Read the model definition and answer for the solid it produces. Units are mm, in the model's axes. Coordinates: 2 decimals unless noted, no trailing zeros. Write each loop counter-clockwise with the first axis right and the second up, starting at its lowest first coordinate (ties: lowest second). Pieces come first, ordered by that corner, then holes.
(1) Straight lines are drawn through the part: line 1 along X through (y, z) = (-19, 14.25); line 2 along Y through (x, z) = (100.5, 24.25). For each, find the intervals that lie inside material, in ascending order.
(2) The part is cut by section B-B, the plane x = 265. Determine the outline of the cut face in (y, z), and give its area (3 significant figures).
(3) The part is cut by section A-A, the plane y = 456.5. Determine the outline of the cut face in (x, z).
(4) The part is cut by section C-C, the plane z = 4.75. Determine the outline of the cut face in (x, y).
```python
from build123d import *

# Parameters (mm, degrees)
CROQUIS1_W              = 1220
CROQUIS1_H              = 2440
CROQUIS1_W_2            = 1118.4
CROQUIS1_H_2            = 2338.4
SALIENTE_EXTRUIR1_DEPTH = 25.4
CROQUIS2_W              = 50.8
CROQUIS2_H              = 2338.4
SALIENTE_EXTRUIR2_DEPTH = 25.4


with BuildPart() as part:
    # Croquis1 → Saliente-Extruir1 (new body)
    with BuildSketch(Plane.XY):
        Rectangle(CROQUIS1_W, CROQUIS1_H)
        Rectangle(CROQUIS1_W_2, CROQUIS1_H_2, mode=Mode.SUBTRACT)
    extrude(amount=SALIENTE_EXTRUIR1_DEPTH)

    # Croquis2 → Saliente-Extruir2 (add)
    with BuildSketch(Plane.XY.offset(25.4)):
        with Locations((-186.4, 0)):
            Rectangle(CROQUIS2_W, CROQUIS2_H)
        with Locations((186.4, 0)):
            Rectangle(CROQUIS2_W, CROQUIS2_H)
    extrude(amount=-SALIENTE_EXTRUIR2_DEPTH)


solid = part.part
```
Computed:
1. line 1: x = -610 to -559.2, -211.8 to -161, 161 to 211.8, 559.2 to 610
1. line 2: y = -1220 to -1169.2, 1169.2 to 1220
2. outline: (-1220, 0) - (-1169.2, 0) - (-1169.2, 25.4) - (-1220, 25.4) - close; (1169.2, 0) - (1220, 0) - (1220, 25.4) - (1169.2, 25.4) - close
2. area: 2,580 mm2
3. outline: (-610, 0) - (-559.2, 0) - (-559.2, 25.4) - (-610, 25.4) - close; (-211.8, 0) - (-161, 0) - (-161, 25.4) - (-211.8, 25.4) - close; (161, 0) - (211.8, 0) - (211.8, 25.4) - (161, 25.4) - close; (559.2, 0) - (610, 0) - (610, 25.4) - (559.2, 25.4) - close
4. outline: (-610, -1220) - (610, -1220) - (610, 1220) - (-610, 1220) - close; hole (-559.2, -1169.2) - (-211.8, -1169.2) - (-211.8, 1169.2) - (-559.2, 1169.2) - close; hole (-161, -1169.2) - (161, -1169.2) - (161, 1169.2) - (-161, 1169.2) - close; hole (211.8, -1169.2) - (559.2, -1169.2) - (559.2, 1169.2) - (211.8, 1169.2) - close
